Design review of the part built by this model. Coordinates are the model's own, in mm. A direction names the side the tool comes from. Round coordinates to 2 decimals unless told otherwise and drop trailing zeros. Loops run counter-clockwise (first coordinate to the right, second up) from the corner with the lowest first, then second, coordinate; pieces in that order, holes last. Notation, with made-up numbers: (-3, 23.25) - (17, 23.25) arc R24 cw to (17, 38.25) - close; hole circle Ø8 at (-1.5, -7). An arc over 180 degrees is marked (long way). Return JSON: item names as keys, results as strings. Group by question number.
(1) We need section D-D, the plane y = -3. Write out the cut boundary in (x, z), and give its area (3 significant figures).
(2) For faces 1 (the flat face through (0, -1.5, -0.19)), 2 (the cylindrical face through (2.278, -0.796, 0.003)), list the 3-axis set-ups (+Z, -Z, +X, -X, +Y, -Y) from which the entire face can be reached by the end or side of a thin tool; tool diameter is ignored.
(3) We need section B-B, the plane x = 1.5. Write out the cut boundary in (y, z), and give its area (3 significant figures).
(4) Wall thickness on L1, parallel to X at y = -1.75, z = 0.15; L2, parallel to X at y = -1.25, z = -0.15; L3, parallel to X at y = 0.75, z = 0: over which ranges is each line inside the solid? List them lowest first. Write a range as [from, to].
(5) The part is to be moulded in two halves that separate along Y. For faces 3 (the cylindrical face through (0.067, -3.174, 0.003)), 4 (the flat face through (0, -1.5, 0.19)), 5 (the cylindrical face through (-2.29, -0.76, 0)), say which applies: pulls with the +Y half, pulls with the -Y half, needs draft (parallel to the pull), parting line crosses it, or undercut.
from build123d import *

# Parameters (mm, degrees)
SKETCH1_R           = 3.175
SKETCH1_R_2         = 1.190625
BOSS_EXTRUDE1_DEPTH = 0.1905
CUT_EXTRUDE1_DEPTH  = 1.381
CUT_EXTRUDE2_DEPTH  = 1.381
FILLET1_R           = 0.381
FILLET1_2_R         = 0.127


with BuildPart() as part:
    # Sketch1 → Boss-Extrude1 (new body, symmetric)
    with BuildSketch(Plane.XY):
        Circle(SKETCH1_R)
        Circle(SKETCH1_R_2, mode=Mode.SUBTRACT)
    extrude(amount=BOSS_EXTRUDE1_DEPTH, both=True)

    # Sketch2 → Cut-Extrude1 (cut, through all)
    with BuildSketch(Plane.XY.offset(0.1905)):
        Polygon((-0.635, 0.3107001), (0.635, 0.3107001), (1.27, 3.175), (-1.27, 3.175), align=None)
    extrude(amount=-CUT_EXTRUDE1_DEPTH, mode=Mode.SUBTRACT)

    # Sketch3 → Cut-Extrude2 (cut, through all)
    with BuildSketch(Plane.XY.offset(0.1905)):
        with BuildLine():
            Line((0.50292, -1.079193849), (1.019518005, -2.187041846))
            ThreePointArc((1.019518005, -2.187041846), (2.284896317, -0.775769179), (2.14035714, 1.114199404))
            Line((2.14035714, 1.114199404), (1.056097273, 0.549769443))
            ThreePointArc((1.056097273, 0.549769443), (1.127392596, -0.382849611), (0.50292, -1.079193849))
        make_face()
        with BuildLine():
            Line((-1.056097273, 0.549769443), (-2.14035714, 1.114199404))
            ThreePointArc((-2.14035714, 1.114199404), (-2.284896317, -0.775769179), (-1.019518005, -2.187041846))
            Line((-1.019518005, -2.187041846), (-0.50292, -1.079193849))
            ThreePointArc((-0.50292, -1.079193849), (-1.127392596, -0.382849611), (-1.056097273, 0.549769443))
        make_face()
    extrude(amount=-CUT_EXTRUDE2_DEPTH, mode=Mode.SUBTRACT)

    # Fillet1
    fillet1_edges = [part.edges().sort_by_distance(p)[0] for p in [
        (-1.216302436, 2.932785942, 0),
        (-2.14035714, 1.114199404, 0),
        (-1.019518005, -2.187041846, 0),
        (-0.50292, -1.079193849, 0),
        (0.50292, -1.079193849, 0),
        (1.019518005, -2.187041846, 0),
        (2.14035714, 1.114199404, 0),
    ]]
    fillet(fillet1_edges, radius=FILLET1_R)

    # Fillet1 2
    fillet1_2_edges = [part.edges().sort_by_distance(p)[0] for p in [
        (1.216302436, 2.932785942, 0),
        (-0.767848913, 0.909942821, 0),
        (-1.056097273, 0.549769443, 0),
        (1.056097273, 0.549769443, 0),
        (0.767848913, 0.909942821, 0),
    ]]
    fillet(fillet1_2_edges, radius=FILLET1_2_R)


solid = part.part
Solutions:
{
 "1": {"outline": "(-1.04, -0.19) - (1.04, -0.19) - (1.04, 0.19) - (-1.04, 0.19) - close", "area": "0.792 mm^2"},
 "2": {"face 1": "-Z, +X, -X, +Y, -Y", "face 2": "+Z, -Z"},
 "3": {"outline": "(-2.8, -0.19) - (-1.89, -0.19) - (-1.89, 0.19) - (-2.8, 0.19) - close; (0.78, -0.19) - (2.8, -0.19) - (2.8, 0.19) - (0.78, 0.19) - close", "area": "1.11 mm^2"},
 "4": {"L1": "[-2.65, -1.66], [-0.82, 0.82], [1.66, 2.65]", "L2": "[-2.92, -2.06], [-0.54, 0.54], [2.06, 2.92]", "L3": "[-3.09, -2.29], [-1.44, -0.92], [0.92, 1.44], [2.29, 3.09]"},
 "5": {"face 3": "parting line crosses it", "face 4": "needs draft", "face 5": "undercut"}
}
